For this review, take the finished solid that the model builds, in its own axes (mm). A direction names the side the tool comes from. Give positions to 0.01 mm unless a question says otherwise; leave off trailing zeros. Order: outer loops, then holes, each group sorted by start corner. A loop starts at its lowest first (then second) coordinate and runs counter-clockwise, first axis right, second up.
from build123d import *

# Parameters (mm, degrees)
BOSS_EXTRUDE1_DEPTH = 5
BOSS_EXTRUDE2_DEPTH = 15
SKETCH3_W           = 14
SKETCH3_H           = 4
CUT_EXTRUDE1_DEPTH  = 15


with BuildPart() as part:
    # Sketch1 → Boss-Extrude1 (new body)
    with BuildSketch(Plane(origin=(0, 0, 0), x_dir=(1, 0, 0), z_dir=(0, 1, 0))):
        with BuildLine():
            Line((-15, -57), (15, -57))
            ThreePointArc((15, -57), (44.69848481, -44.69848481), (57, -15))
            Line((57, -15), (57, 15))
            ThreePointArc((57, 15), (44.69848481, 44.69848481), (15, 57))
            Line((15, 57), (-15, 57))
            ThreePointArc((-15, 57), (-44.69848481, 44.69848481), (-57, 15))
            Line((-57, 15), (-57, -15))
            ThreePointArc((-57, -15), (-44.69848481, -44.69848481), (-15, -57))
        make_face()
    extrude(amount=BOSS_EXTRUDE1_DEPTH)

    # Sketch2 → Boss-Extrude2 (add)
    with BuildSketch(Plane(origin=(0, 5, 0), x_dir=(1, 0, 0), z_dir=(0, 1, 0))):
        with BuildLine():
            Line((57, -15), (57, 15))
            ThreePointArc((57, 15), (44.69848481, 44.69848481), (15, 57))
            Line((15, 57), (-15, 57))
            ThreePointArc((-15, 57), (-44.69848481, 44.69848481), (-57, 15))
            Line((-57, 15), (-57, -15))
            ThreePointArc((-57, -15), (-44.69848481, -44.69848481), (-15, -57))
            Line((-15, -57), (15, -57))
            ThreePointArc((15, -57), (44.69848481, -44.69848481), (57, -15))
        make_face()
        with BuildLine():
            Line((-53, 15), (-53, -15))
            ThreePointArc((-53, -15), (-41.870057685, -41.870057685), (-15, -53))
            Line((-15, -53), (15, -53))
            ThreePointArc((15, -53), (41.870057685, -41.870057685), (53, -15))
            Line((53, -15), (53, 15))
            ThreePointArc((53, 15), (41.870057685, 41.870057685), (15, 53))
            Line((15, 53), (-15, 53))
            ThreePointArc((-15, 53), (-41.870057685, 41.870057685), (-53, 15))
        make_face(mode=Mode.SUBTRACT)
    extrude(amount=BOSS_EXTRUDE2_DEPTH)

    # Sketch3 → Cut-Extrude1 (cut)
    with BuildSketch(Plane(origin=(0, 20, 0), x_dir=(1, 0, 0), z_dir=(0, 1, 0))):
        with Locations((0, -55)):
            Rectangle(SKETCH3_W, SKETCH3_H)
    extrude(amount=-CUT_EXTRUDE1_DEPTH, mode=Mode.SUBTRACT)


solid = part.part
1) To check wall thickness, follow line 1 (X direction, y = 10.75, z = -16.5); line 2 (Y direction, x = -28, z = -22.5); line 3 (Z direction, x = -46, y = 7.75). State the ranges of each line that lie inside material, in increasing order.
Answer sheet:
line 1: x = -56.97 to -52.97, 52.97 to 56.97
line 2: y = 0 to 5
line 3: z = -43.34 to -36.98, 36.98 to 43.34
2) Draft analysis for pull direction X (two halves, no side actions). For faces 1 (the face through (-57, 10, 0)), 2 (the face through (-53, 12, 0)), 3 (the face through (0, 10, -57)), 4 (the face through (0, 12, -53)), state which applies: +X half, -X half, draft (parallel to the pull), parting line (faces both ways), or undercut.
Answer sheet:
face 1: -X half
face 2: undercut
face 3: draft
face 4: undercut
3) We need section C-C on z = 9.5. Give the boundary of the cut face in (x, y).
Answer sheet:
outline: (-57, 0) - (57, 0) - (57, 20) - (53, 20) - (53, 5) - (-53, 5) - (-53, 20) - (-57, 20) - close
4) We need section A-A on y = 14. Give the boundary of the cut face in (x, z).
Answer sheet:
outline: (-57, -15) arc R42 ccw to (-15, -57) - (15, -57) arc R42 ccw to (57, -15) - (57, 15) arc R42 ccw to (15, 57) - (7, 57) - (7, 53) - (15, 53) arc R38 cw to (53, 15) - (53, -15) arc R38 cw to (15, -53) - (-15, -53) arc R38 cw to (-53, -15) - (-53, 15) arc R38 cw to (-15, 53) - (-7, 53) - (-7, 57) - (-15, 57) arc R42 ccw to (-57, 15) - close
5) We need section D-D on x = -2.5. Give the boundary of the cut face in (y, z).
Answer sheet:
outline: (0, -57) - (20, -57) - (20, -53) - (5, -53) - (5, 57) - (0, 57) - close
6) Clearance check with flat-ended pins moving along their axes: pin 1 (5 mm diameter, centred on x = -34.5, y = 16.5, fed in from +Z); pin 2 (1.2 mm diameter, centred on y = 13, z = 54.5, fed in from +X); pin 3 (8 mm diameter, centred on x = -45.5, z = -1.5, fed in from +Y). State where each tip first meets the part, or that it passes through.
Answer sheet:
pin 1: stops at z = 53.41
pin 2: stops at x = 30.84
pin 3: stops at y = 5
7) We need section B-B on x = 10. Give the boundary of the cut face in (y, z), then the cut area to 3 significant figures.
Answer sheet:
outline: (0, -57) - (20, -57) - (20, -53) - (5, -53) - (5, 53) - (20, 53) - (20, 57) - (0, 57) - close
area: 690 mm2
8) Tool access review of faces 5 (the face through (11, 12, 53)), 6 (the face through (-7, 13, 55)), 7 (the face through (-44.37, 9.86, -45.023)): name each direction out of +Z, -Z, +X, -X, +Y, -Y from which nothing blocks a thin tool from reaching the whole face with its end or side.
Answer sheet:
face 5: +Y
face 6: +Z, +Y
face 7: -Z, -X, +Y, -Y
